Build history of the part. All positions in model axes, mm. A direction names the side the tool comes from. Round coordinates to 2 decimals unless told otherwise and drop trailing zeros. Write each loop counter-clockwise with the first axis right and the second up, starting at its lowest first coordinate (ties: lowest second). Pieces come first, ordered by that corner, then holes.
1) Flat gauge pins, fed straight in: pin 1 (6 mm diameter, centred on x = 17, z = -78.5, fed in from +Y); pin 2 (12 mm diameter, centred on x = 8, y = -4.5, fed in from -Z); pin 3 (3 mm diameter, centred on x = 3.5, z = -29.5, fed in from -Y); pin 4 (10 mm diameter, centred on x = -13.5, z = 2, fed in from +Y). Where does each tip first touch, or does it go through?
2) Saw through at A-A (y = 0). Write the cut outline in (x, z).
3) Which spindle directions (+Z, -Z, +X, -X, +Y, -Y) get a long thin tool onto all of the face, cutting with end or side? Do faces 4 (the cylindrical face through (19.5, 0.2, -42.8)), 5 (the cylindrical face through (-19.5, -0.2, -42.8)), 6 (the flat face through (0, 14, 0)). Say none if no direction does.
4) Saw through at D-D (z = -67). Write the cut outline in (x, y), plus the area to 3 significant figures.
5) Pull direction Y, two halves, no side cores. Call faces 1 (the flat face through (0, 11.5, -46)), 2 (the flat face through (0, 0, 12.6)), 3 (the flat face through (0, -20.333, 19)): +Y half, -Y half, draft (parallel to the pull), parting line (faces both ways), or undercut.
6) Wall check: probe 1 along Y at (x, z) = (0, 26.25); probe 2 along Z at (x, y) = (1, 12.5); probe 3 along Z at (x, y) = (-14, -17.5). Give the ranges that are in metal, low to high.
7) Saw through at C-C (x = 9). Write the cut outline in (y, z), plus the area to 3 significant figures.
8) Saw through at B-B (z = 18.5). Write the cut outline in (x, y), plus the area to 3 significant figures.
from build123d import *

# Parameters (mm, degrees)
F1_DEPTH = 38
F2_R     = 20.15
F3_DEPTH = 25.4
F5_DEPTH = 93
F7_DEPTH = 31.834163


with BuildPart() as f1:
    # F0 (on Top) → F1 (new body)
    with BuildSketch(Plane.XY):
        with BuildLine():
            Line((10.75, 20.333163), (-10.75, 20.333163))
            ThreePointArc((-10.75, 20.333163), (-23, 0), (-10.75, -20.333163))
            Line((-10.75, -20.333163), (10.75, -20.333163))
            ThreePointArc((10.75, -20.333163), (23, 0), (10.75, 20.333163))
        make_face()
    extrude(amount=F1_DEPTH)

    # F2 (on face) → F3 (cut)
    with BuildSketch(Plane.XY.offset(38)):
        Circle(F2_R)
    extrude(amount=-F3_DEPTH, mode=Mode.SUBTRACT)

    # F4 (on face) → F5 (join)
    with BuildSketch(Plane(origin=(0, 0, 0), x_dir=(1, 0, 0), z_dir=(0, 0, -1))):
        with BuildLine():
            Line((15.748016, 11.5), (-15.748016, 11.5))
            ThreePointArc((-15.748016, 11.5), (-19.5, 0), (-15.748016, -11.5))
            Line((-15.748016, -11.5), (15.748016, -11.5))
            ThreePointArc((15.748016, -11.5), (19.5, 0), (15.748016, 11.5))
        make_face()
    extrude(amount=F5_DEPTH)

    # F6 (on face) → F7 (cut, through all)
    with BuildSketch(Plane.XZ.offset(11.5)):
        with BuildLine():
            ThreePointArc((-15.748016, -86.763055), (-19.645798, -81.960042), (-22.122635, -76.291981))
            Line((-22.122635, -76.291981), (-44.180881, -110.498317))
            Line((-44.180881, -110.498317), (51.086351, -107.824139))
            Line((51.086351, -107.824139), (22.594881, -74.29783))
            ThreePointArc((22.594881, -74.29783), (20.159114, -81.072945), (15.748016, -86.763055))
            Line((15.748016, -86.763055), (15.748016, -93))
            Line((15.748016, -93), (0, -93))
            Line((0, -93), (-15.748016, -93))
            Line((-15.748016, -93), (-15.748016, -86.763055))
        make_face()
        with BuildLine():
            ThreePointArc((15.748016, -86.763055), (8.469054, -91.383992), (0, -93))
            Line((0, -93), (15.748016, -93))
            Line((15.748016, -93), (15.748016, -86.763055))
        make_face()
        with BuildLine():
            ThreePointArc((0, -93), (-8.469054, -91.383992), (-15.748016, -86.763055))
            Line((-15.748016, -86.763055), (-15.748016, -93))
            Line((-15.748016, -93), (0, -93))
        make_face()
    extrude(amount=-F7_DEPTH, mode=Mode.SUBTRACT)


solid = f1.part
Evaluation:
1. pin 1: stops at y = 11.5
1. pin 2: stops at z = -92.91
1. pin 3: stops at y = -11.5
1. pin 4: stops at y = 20.33
2. outline: (-23, 0) - (-19.5, 0) - (-19.5, -82.2) arc R23 ccw to (-15.75, -86.76) arc R23 ccw to (0, -93) arc R23 ccw to (15.75, -86.76) arc R23 ccw to (19.5, -82.2) - (19.5, 0) - (23, 0) - (23, 38) - (20.15, 38) - (20.15, 12.6) - (-20.15, 12.6) - (-20.15, 38) - (-23, 38) - close
3. face 4: -Z, +X
3. face 5: -Z, -X
3. face 6: -Z
4. outline: (-15.75, -11.5) - (15.75, -11.5) arc R19.5 ccw to (15.75, 11.5) - (-15.75, 11.5) arc R19.5 ccw to start
4. area: 842 mm2
5. face 1: +Y half
5. face 2: undercut
5. face 3: -Y half
6. probe 1: y = -20.33 to -20.15, 20.15 to 20.33
6. probe 2: z = 0 to 12.6
6. probe 3: z = 0 to 38
7. outline: (-20.33, 0) - (-11.5, 0) - (-11.5, -91.17) - (11.5, -91.17) - (11.5, 0) - (20.33, 0) - (20.33, 38) - (18.03, 38) - (18.03, 12.6) - (-18.03, 12.6) - (-18.03, 38) - (-20.33, 38) - close
7. area: 2,730 mm2
8. outline: (-10.75, -20.33) - (10.75, -20.33) arc R23 ccw to (10.75, 20.33) - (-10.75, 20.33) arc R23 ccw to start; hole circle Ø40.3 at (0, 0)
8. area: 309 mm2
